from build123d import *

# Parameters (mm, degrees)
SKETCH1_W           = 125
SKETCH1_H           = 66
BOSS_EXTRUDE1_DEPTH = 155
FILLET1_R           = 2
SKETCH7_R           = 1.4
CUT_EXTRUDE4_DEPTH  = 15
SKETCH4_W           = 121
SKETCH4_H           = 151
CUT_EXTRUDE5_DEPTH  = 64
SKETCH8_W           = 101
SKETCH8_H           = 64.031377795
CUT_EXTRUDE6_DEPTH  = 64


with BuildPart() as part:
    # Sketch1 → Boss-Extrude1 (new body)
    with BuildSketch(Plane.XY):
        with Locations((-19.516389056, 19.409080835)):
            Rectangle(SKETCH1_W, SKETCH1_H)
    extrude(amount=BOSS_EXTRUDE1_DEPTH)

    # Fillet1
    fillet1_edges = [part.edges().sort_by_distance(p)[0] for p in [
        (-82.016389056, 52.409080835, 77.5),
        (42.983610944, 52.409080835, 77.5),
        (42.983610944, -13.590919165, 77.5),
        (-82.016389056, -13.590919165, 77.5),
    ]]
    fillet(fillet1_edges, radius=FILLET1_R)

    # Sketch7 → Cut-Extrude4 (cut)
    with BuildSketch(Plane.XY.offset(155)):
        with Locations((-75.016389056, 45.409080835)):
            Circle(SKETCH7_R)
        with Locations((-75.016389056, -6.590919165)):
            Circle(SKETCH7_R)
        with Locations((35.983610944, -6.590919165)):
            Circle(SKETCH7_R)
        with Locations((35.983610944, 45.409080835)):
            Circle(SKETCH7_R)
    extrude(amount=-CUT_EXTRUDE4_DEPTH, mode=Mode.SUBTRACT)

    # Sketch4 → Cut-Extrude5 (cut)
    with BuildSketch(Plane(origin=(0, 52.409080835, 0), x_dir=(1, 0, 0), z_dir=(0, 1, 0))):
        with Locations((-19.516389056, -77.5)):
            Rectangle(SKETCH4_W, SKETCH4_H)
    extrude(amount=-CUT_EXTRUDE5_DEPTH, mode=Mode.SUBTRACT)

    # Sketch8 → Cut-Extrude6 (cut)
    with BuildSketch(Plane.XY.offset(155)):
        with Locations((-19.516389056, 20.424769732)):
            Rectangle(SKETCH8_W, SKETCH8_H)
    extrude(amount=-CUT_EXTRUDE6_DEPTH, mode=Mode.SUBTRACT)


solid = part.part
CAD build for the part. Positions are in the model's coordinates, mm. A direction names the side the tool comes from. Coordinates: 2 decimals unless noted, no trailing zeros. Write each loop counter-clockwise with the first axis right and the second up, starting at its lowest first coordinate (ties: lowest second). Pieces come first, ordered by that corner, then holes. Notation, with made-up numbers: (-27.75, -1) - (22.25, -1) arc R12 cw to (22.25, 5) - close; hole circle Ø11 at (-34.75, 53.25). An arc over 180 degrees is marked (long way). Use a Markdown table: item, result. Add a question column.
Item 1: Band-saw the part on A-A, the plane y = 2. Give the cut face in (x, z).
Item 2: Band-saw the part on C-C, the plane x = 10. Give the cut face in (y, z), and give its area (3 significant figures).
Item 3: Drill centre lines: L1, parallel to Z at x = 34.5, y = 34; L2, parallel to X at y = 35, z = 46.5; L3, parallel to Y at x = 22, z = 41. Where is each one in solid material? Low to high. Write a range as from..to.
Item 4: Mould opens along X. For faces 1 (the face through (-20, -13.591, 76)), 2 (the face through (-80.016, 21, 79)), 3 (the face through (-20, -11.591, 80)), 4 (the face through (42.984, 19, 76)) say: pulls with the +X half, pulls with the -X half, needs draft (parallel to the pull), parting line crosses it, or undercut.
Item 5: 3-axis set-ups, long thin cutter, end or side, ignore diameter. For faces 5 (the face through (-82.016, 19, 76)), 6 (the face through (-75, 21, 153)): which of +Z, -Z, +X, -X, +Y, -Y reach the whole face in a straight line?
Item 6: Band-saw the part on B-B, the plane z = 85. Give the cut face in (x, y).
Item 7: Flat gauge pins, fed straight in: pin 1 (5 mm diameter, centred on x = -75, y = 28, fed in from -Z); pin 2 (1.7 mm diameter, centred on x = -75.02, y = 45.41, fed in from +Z); pin 3 (4 mm diameter, centred on x = -37, z = 95.5, fed in from +Y). Where does each tip first touch, or does it go through?
Numbers:
| question | item | result |
|---|---|---|
| 1 | outline | (-82.02, 0) - (42.98, 0) - (42.98, 155) - (30.98, 155) - (30.98, 153) - (40.98, 153) - (40.98, 2) - (-80.02, 2) - (-80.02, 153) - (-70.02, 153) - (-70.02, 155) - (-82.02, 155) - close |
| 2 | outline | (-13.59, 0) - (52.41, 0) - (52.41, 2) - (-11.59, 2) - (-11.59, 155) - (-13.59, 155) - close |
| 2 | area | 438 mm2 |
| 3 | L1 | 0..2, 153..155 |
| 3 | L2 | -82.02..-80.02, 40.98..42.98 |
| 3 | L3 | -13.59..-11.59 |
| 4 | face 1 | needs draft |
| 4 | face 2 | undercut |
| 4 | face 3 | undercut |
| 4 | face 4 | pulls with the +X half |
| 5 | face 5 | +Z, -Z, -X, +Y, -Y |
| 5 | face 6 | +Y |
| 6 | outline | (-82.02, -11.59) arc R2 ccw to (-80.02, -13.59) - (40.98, -13.59) arc R2 ccw to (42.98, -11.59) - (42.98, 50.41) arc R2 ccw to (40.98, 52.41) - (40.98, -11.59) - (-80.02, -11.59) - (-80.02, 52.41) arc R2 ccw to (-82.02, 50.41) - close |
| 7 | pin 1 | z = 0 |
| 7 | pin 2 | z = 2 |
| 7 | pin 3 | y = -11.59 |
